Design review of the part shown in the three views and the two pictorial views. Dimensions are in mm from the part's minimum x, y and z. Give positions to 0.01 mm unless a question says otherwise; leave off trailing zeros. Loops run counter-clockwise (first coordinate to the right, second up) from the corner with the lowest first, then second, coordinate; pieces in that order, holes last.
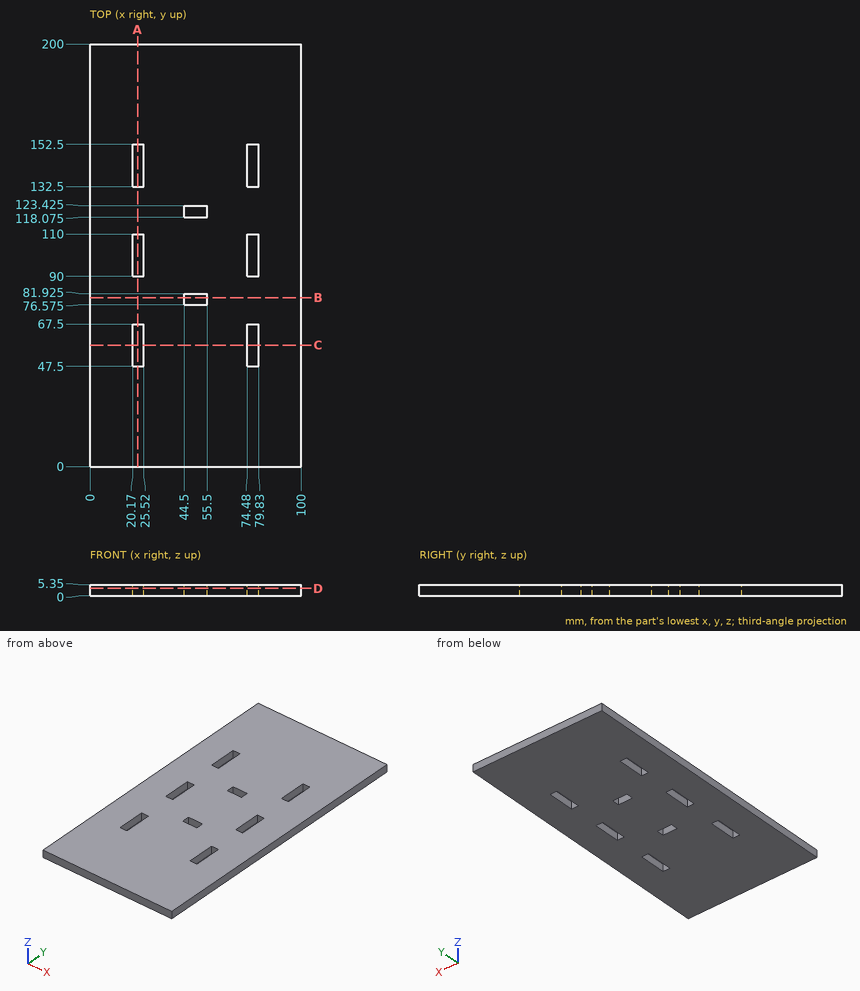
Q1. Take a section at A-A (x = 22.5). Give the boundary of the cut face in (y, z), plus the area to 3 significant figures.
Results:
outline: (0, 0) - (47.5, 0) - (47.5, 5.35) - (0, 5.35) - close; (67.5, 0) - (90, 0) - (90, 5.35) - (67.5, 5.35) - close; (110, 0) - (132.5, 0) - (132.5, 5.35) - (110, 5.35) - close; (152.5, 0) - (200, 0) - (200, 5.35) - (152.5, 5.35) - close
area: 749 mm2
Q2. Take a section at D-D (z = 3.65). Give the number of separate pieces and of enclosed holes in the cut face, plus the area to 3 significant figures.
Results:
separate pieces: 1
enclosed holes: 8
area: 19,200 mm2
Q3. Take a section at B-B (y = 80). Give the boundary of the cut face in (x, z), plus the area to 3 significant figures.
Results:
outline: (0, 0) - (44.5, 0) - (44.5, 5.35) - (0, 5.35) - close; (55.5, 0) - (100, 0) - (100, 5.35) - (55.5, 5.35) - close
area: 476 mm2
Q4. Take a section at C-C (y = 57.5). Give the boundary of the cut face in (x, z).
Results:
outline: (0, 0) - (20.17, 0) - (20.17, 5.35) - (0, 5.35) - close; (25.52, 0) - (74.48, 0) - (74.48, 5.35) - (25.52, 5.35) - close; (79.83, 0) - (100, 0) - (100, 5.35) - (79.83, 5.35) - close
Q5. Wall thickness on line 1 (X direction, y = 136, z = 0.9); line 2 (Y direction, x = 79.5, z = 1.9); line 3 (Y direction, x = 52.5, z = 4.05) (3 decimals): over which ranges is each line inside the solid? List them lowest first.
Results:
line 1: x = 0 to 20.17, 25.52 to 74.48, 79.83 to 100
line 2: y = 0 to 47.5, 67.5 to 90, 110 to 132.5, 152.5 to 200
line 3: y = 0 to 76.575, 81.925 to 118.075, 123.425 to 200
